Input: part model. Units: mm. Frame: model coordinates. Face numbers are marked on the shaded views. Coordinates: 2 decimals unless noted, no trailing zeros. Loops run counter-clockwise (first coordinate to the right, second up) from the corner with the lowest first, then second, coordinate; pieces in that order, holes last.
Item 1: Contact query for flat-ended pins moving along their axis: P1, Ø5, axis at x = 0, y = 0, coming from the +Z side; P2, Ø1, axis at y = 6, z = -3, coming from the +X side. Output: stop coordinate, or through.
Item 2: Pull-direction query (Y, two-part tool) for the marked faces 1, 2 and 3; classes: released by +Y, released by -Y, zero draft, split by the parting line, or undercut.
Item 3: Ray query, line 1 along X through (y, z) = (-3, -2.8); line 2 along Y through (x, z) = (0, -3.95); line 3 along Y through (x, z) = (3, -1.5). Return the intervals inside material, ascending.
Item 4: Section A-A on z = -1.1. Return loops of the section in (x, y), and give its area (3 significant figures).
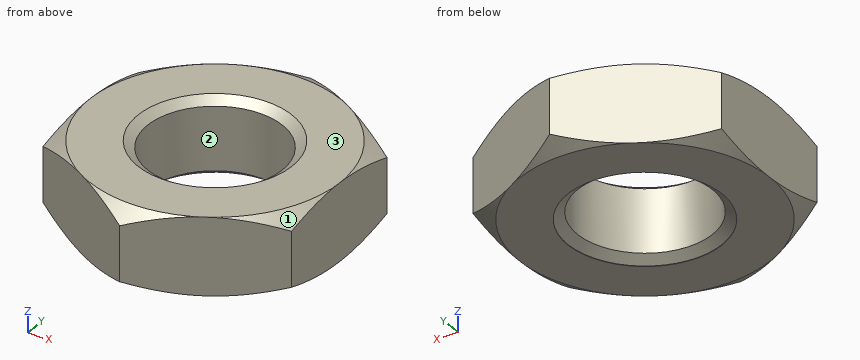
```python
from build123d import *

# Parameters (mm, degrees)
BASENUTSKE_R  = 3.5
BASENUT_DEPTH = 4


# Read off the part's stored shape, not the designer's step: ThreadSchematic
with BuildPart() as part:
    # BaseNutSke → BaseNut (new body)
    with BuildSketch(Plane.XY):
        Polygon((6.5, 3.75277675), (6.5, -3.75277675), (0, -7.505553499), (-6.5, -3.75277675), (-6.5, 3.75277675), (0, 7.505553499), align=None)
        Circle(BASENUTSKE_R, mode=Mode.SUBTRACT)
    extrude(amount=-BASENUT_DEPTH)

    # Sketch3 → Double-Chamfer (revolve, cut)
    with BuildSketch(Plane(origin=(0, 0, 0), x_dir=(0, 0, -1), z_dir=(1, 0, 0))):
        Polygon((4, 6.5), (3.419443416, 7.505553499), (3.419443416, 17.505553499), (14, 17.505553499), (14, 6.5), align=None)
        Polygon((0.580556584, 17.505553499), (-10, 17.505553499), (-10, 6.5), (0, 6.5), (0.580556584, 7.505553499), align=None)
    revolve(axis=Axis((0, 0, 0), (0, 0, -1)), mode=Mode.SUBTRACT)

    # ThreadSchematic outline → ThreadSchematic (revolve, cut)
    with BuildSketch(Plane.XZ):
        Polygon((3.5, 0), (3.5, -0.350103769), (4, 0), align=None)
        Polygon((4, -3.9746), (3.5, -3.624496231), (3.5, -4), (4, -4), align=None)
    revolve(axis=Axis((0, 0, 0), (0, 0, 1)), mode=Mode.SUBTRACT)


solid = part.part
```
Results found:
1. P1: passes through
1. P2: stops at x = 3.47
2. face 1: released by -Y
2. face 2: undercut
2. face 3: zero draft
3. line 1: x = -6.5 to -1.8, 1.8 to 6.5
3. line 2: y = -6.59 to -3.96, 3.96 to 6.59
3. line 3: y = -5.77 to -1.8, 1.8 to 5.77
4. outline: (-6.5, -3.75) - (0, -7.51) - (6.5, -3.75) - (6.5, 3.75) - (0, 7.51) - (-6.5, 3.75) - close; hole circle Ø7 at (0, 0)
4. area: 108 mm2
